Build history of the part. All positions in model axes, mm. A direction names the side the tool comes from. Give positions to 0.01 mm unless a question says otherwise; leave off trailing zeros. Loops run counter-clockwise (first coordinate to the right, second up) from the corner with the lowest first, then second, coordinate; pieces in that order, holes last. Notation, with made-up numbers: (-25.5, -30.5) -> (-9.5, -30.5) arc R13 ccw to (-9.5, -16.5) -> close; hole circle Ø6 at (13.5, -37). An arc over 180 degrees is marked (long way). Answer as a JSON object with one key per item and string values. Group by question number.
from build123d import *

# Parameters (mm, degrees)
SKETCH1_R                       = 4
BOSS_EXTRUDE1_DEPTH             = 45
SKETCH2_R                       = 1.625
BOSS_EXTRUDE2_DEPTH             = 2
FILLET1_R                       = 1
FILLET1_OF_MIRROR1_R            = 1
BOSS_EXTRUDE3_REACH             = 49.339
BOSS_EXTRUDE3_DIRECTION_2_REACH = 49.339
SKETCH5_W                       = 68.734952121
SKETCH5_H                       = 6.985
BOSS_EXTRUDE4_DEPTH             = 3.25
FILLET2_R                       = 3.175
FILLET3_R                       = 10
BOSS_EXTRUDE5_DEPTH             = 36.449
SKETCH7_W                       = 19.05
SKETCH7_H                       = 25.4
CUT_EXTRUDE1_DEPTH              = 33.782
FILLET4_R                       = 2
CUT_EXTRUDE2_DEPTH              = 134.693288074
CUT_EXTRUDE3_DEPTH              = 99.825981407
CUT_EXTRUDE3_DEPTH_BACK         = 99.825981407
SKETCH13_R                      = 1.625
SKETCH14_W                      = 22.869052137
SKETCH14_H                      = 20
CUT_EXTRUDE4_DEPTH              = 134.693288074
FILLET5_R                       = 1


with BuildPart() as part:
    # Sketch1 → Boss-Extrude1 (new, symmetric)
    with BuildSketch(Plane.XY):
        with Locations(Location((0, 0, 0), (0, 0, 180))):
            Circle(SKETCH1_R)
    extrude(amount=BOSS_EXTRUDE1_DEPTH, both=True)

    # Sketch2 → Boss-Extrude2 (add)
    with BuildSketch(Plane.XY.offset(45)):
        Circle(SKETCH2_R)
    boss_extrude2 = extrude(amount=BOSS_EXTRUDE2_DEPTH)

    # Fillet1
    fillet1_edges = [part.edges().sort_by_distance(p)[0] for p in [
        (-1.625, 0, 47),
    ]]
    fillet(fillet1_edges, radius=FILLET1_R)

    # Mirror1: Boss-Extrude2 across plane
    add(boss_extrude2.mirror(Plane.XY))

    # Fillet1 of Mirror1
    fillet1_of_mirror1_edges = [part.edges().sort_by_distance(p)[0] for p in [
        (-1.625, 0, -47),
    ]]
    fillet(fillet1_of_mirror1_edges, radius=FILLET1_OF_MIRROR1_R)

    # Boss-Extrude3: up to this face of the body (flat: up to its plane)
    boss_extrude3_end = Plane(part.part.faces().sort_by_distance((3.886862915, 0, 45))[0])
    # Sketch3 → Boss-Extrude3 (add, up to the picked face)
    with BuildSketch(Plane.XY, mode=Mode.PRIVATE) as boss_extrude3_sk1:
        Polygon((0, 0), (0, 1.625), (-74.93, 1.625), (-74.93, -1.625), (0, -1.625), align=None)
    boss_extrude3_tool1 = split(extrude(boss_extrude3_sk1.sketch, amount=BOSS_EXTRUDE3_REACH, mode=Mode.PRIVATE), bisect_by=boss_extrude3_end, keep=Keep.BOTH, mode=Mode.PRIVATE)
    add(boss_extrude3_tool1.solids().sort_by(Axis((-37.465, 0, 0), (0, 0, 1)))[0])

    # Boss-Extrude3 direction 2: up to this face of the body (flat: up to its plane)
    boss_extrude3_direction_2_end = Plane(part.part.faces().sort_by_distance((3.886862915, 0, -45))[0])
    # Sketch3 → Boss-Extrude3 direction 2 (add, up to the picked face)
    with BuildSketch(Plane.XY, mode=Mode.PRIVATE) as boss_extrude3_direction_2_sk1:
        Polygon((0, 0), (0, 1.625), (-74.93, 1.625), (-74.93, -1.625), (0, -1.625), align=None)
    boss_extrude3_direction_2_tool1 = split(extrude(boss_extrude3_direction_2_sk1.sketch, amount=-BOSS_EXTRUDE3_DIRECTION_2_REACH, mode=Mode.PRIVATE), bisect_by=boss_extrude3_direction_2_end, keep=Keep.BOTH, mode=Mode.PRIVATE)
    add(boss_extrude3_direction_2_tool1.solids().sort_by(Axis((-37.465, 0, 0), (0, 0, -1)))[0])

    # Sketch5 → Boss-Extrude4 (add)
    with BuildSketch(Plane(origin=(0, 1.625, 0), x_dir=(1, 0, 0), z_dir=(0, 1, 0))):
        with Locations((-40.56252394, 48.4925)):
            Rectangle(SKETCH5_W, SKETCH5_H)
    boss_extrude4 = extrude(amount=-BOSS_EXTRUDE4_DEPTH)

    # Mirror2: Boss-Extrude4 across plane
    add(boss_extrude4.mirror(Plane.XY))

    # Fillet2
    # the kernel refuses this fillet: 3.175 mm, written as the material it adds along each edge
    with BuildSketch(Plane(origin=(-6.195047879, 1.625, -45), x_dir=(1, 0, 0), z_dir=(0, -1, 0))) as fillet2_piece_1_section:
        with BuildLine():
            CenterArc((FILLET2_R, -FILLET2_R), FILLET2_R, 90, 90)
            Line((0, -FILLET2_R), (0, 0))
            Line((0, 0), (FILLET2_R, 0))
        make_face()
    fillet2_piece_1 = extrude(amount=3.25, mode=Mode.PRIVATE)
    fillet2_piece_1 = fillet2_piece_1 - Plane(origin=(0, 0, -45.745349648), x_dir=(-1, 0, 0), z_dir=(0, 0, 1)) * Cylinder(4, 20, mode=Mode.PRIVATE)
    add(fillet2_piece_1)
    with BuildSketch(Plane(origin=(-6.195047879, 9.5625, -45), x_dir=(1, 0, 0), z_dir=(0, -1, 0))) as fillet2_piece_2_section:
        with BuildLine():
            CenterArc((FILLET2_R, -FILLET2_R), FILLET2_R, 90, 90)
            Line((0, -FILLET2_R), (0, 0))
            Line((0, 0), (FILLET2_R, 0))
        make_face()
    fillet2_piece_2 = extrude(amount=11.1875, mode=Mode.PRIVATE)
    fillet2_piece_2 = split(fillet2_piece_2, bisect_by=Plane(origin=(-3.269448726, 1.625, -44.97522317), z_dir=(0, 1, 0)), keep=Keep.TOP, mode=Mode.PRIVATE)
    fillet2_piece_2 = fillet2_piece_2 & Plane(origin=(0, 0, -44.97522317), x_dir=(-1, 0, 0), z_dir=(0, 0, 1)) * Cylinder(4, 36, mode=Mode.PRIVATE)
    add(fillet2_piece_2)
    with BuildSketch(Plane(origin=(-6.195047879, 1.625, -45), x_dir=(1, 0, 0), z_dir=(0, -1, 0))) as fillet2_piece_3_section:
        with BuildLine():
            CenterArc((FILLET2_R, -FILLET2_R), FILLET2_R, 90, 90)
            Line((0, -FILLET2_R), (0, 0))
            Line((0, 0), (FILLET2_R, 0))
        make_face()
    fillet2_piece_3 = extrude(amount=3.25, mode=Mode.PRIVATE)
    fillet2_piece_3 = fillet2_piece_3 & Plane(origin=(0, 0, -44.99635319), x_dir=(-1, 0, 0), z_dir=(0, 0, 1)) * Cylinder(4, 20, mode=Mode.PRIVATE)
    add(fillet2_piece_3)
    with BuildSketch(Plane(origin=(-6.195047879, 1.625, -45), x_dir=(1, 0, 0), z_dir=(0, -1, 0))) as fillet2_piece_4_section:
        with BuildLine():
            CenterArc((FILLET2_R, -FILLET2_R), FILLET2_R, 90, 90)
            Line((0, -FILLET2_R), (0, 0))
            Line((0, 0), (FILLET2_R, 0))
        make_face()
    fillet2_piece_4 = extrude(amount=11.1875, mode=Mode.PRIVATE)
    fillet2_piece_4 = split(fillet2_piece_4, bisect_by=Plane(origin=(-3.269448726, -1.625, -44.97522317), z_dir=(0, -1, 0)), keep=Keep.TOP, mode=Mode.PRIVATE)
    fillet2_piece_4 = fillet2_piece_4 & Plane(origin=(0, 0, -44.97522317), x_dir=(-1, 0, 0), z_dir=(0, 0, 1)) * Cylinder(4, 36, mode=Mode.PRIVATE)
    add(fillet2_piece_4)
    with BuildSketch(Plane(origin=(-6.195047879, 1.625, 45), x_dir=(1, 0, 0), z_dir=(0, -1, 0))) as fillet2_piece_5_section:
        with BuildLine():
            CenterArc((FILLET2_R, FILLET2_R), FILLET2_R, 180, 90)
            Line((0, FILLET2_R), (0, 0))
            Line((0, 0), (FILLET2_R, 0))
        make_face()
    fillet2_piece_5 = extrude(amount=3.25, mode=Mode.PRIVATE)
    fillet2_piece_5 = fillet2_piece_5 - Plane(origin=(0, 0, 45.745349648), x_dir=(-1, 0, 0), z_dir=(0, 0, 1)) * Cylinder(4, 20, mode=Mode.PRIVATE)
    add(fillet2_piece_5)
    with BuildSketch(Plane(origin=(-6.195047879, 9.5625, 45), x_dir=(1, 0, 0), z_dir=(0, -1, 0))) as fillet2_piece_6_section:
        with BuildLine():
            CenterArc((FILLET2_R, FILLET2_R), FILLET2_R, 180, 90)
            Line((0, FILLET2_R), (0, 0))
            Line((0, 0), (FILLET2_R, 0))
        make_face()
    fillet2_piece_6 = extrude(amount=11.1875, mode=Mode.PRIVATE)
    fillet2_piece_6 = fillet2_piece_6 & Plane(origin=(0, 0, 44.97522317), x_dir=(-1, 0, 0), z_dir=(0, 0, 1)) * Cylinder(4, 36, mode=Mode.PRIVATE)
    fillet2_piece_6 = split(fillet2_piece_6, bisect_by=Plane(origin=(-3.269448726, 1.625, 44.97522317), z_dir=(0, 1, 0)), keep=Keep.TOP, mode=Mode.PRIVATE)
    add(fillet2_piece_6)
    with BuildSketch(Plane(origin=(-6.195047879, 1.625, 45), x_dir=(1, 0, 0), z_dir=(0, -1, 0))) as fillet2_piece_7_section:
        with BuildLine():
            CenterArc((FILLET2_R, FILLET2_R), FILLET2_R, 180, 90)
            Line((0, FILLET2_R), (0, 0))
            Line((0, 0), (FILLET2_R, 0))
        make_face()
    fillet2_piece_7 = extrude(amount=3.25, mode=Mode.PRIVATE)
    fillet2_piece_7 = fillet2_piece_7 & Plane(origin=(0, 0, 44.99635319), x_dir=(-1, 0, 0), z_dir=(0, 0, 1)) * Cylinder(4, 20, mode=Mode.PRIVATE)
    add(fillet2_piece_7)
    with BuildSketch(Plane(origin=(-6.195047879, 1.625, 45), x_dir=(1, 0, 0), z_dir=(0, -1, 0))) as fillet2_piece_8_section:
        with BuildLine():
            CenterArc((FILLET2_R, FILLET2_R), FILLET2_R, 180, 90)
            Line((0, FILLET2_R), (0, 0))
            Line((0, 0), (FILLET2_R, 0))
        make_face()
    fillet2_piece_8 = extrude(amount=11.1875, mode=Mode.PRIVATE)
    fillet2_piece_8 = fillet2_piece_8 & Plane(origin=(0, 0, 44.97522317), x_dir=(-1, 0, 0), z_dir=(0, 0, 1)) * Cylinder(4, 36, mode=Mode.PRIVATE)
    fillet2_piece_8 = split(fillet2_piece_8, bisect_by=Plane(origin=(-3.269448726, -1.625, 44.97522317), z_dir=(0, -1, 0)), keep=Keep.TOP, mode=Mode.PRIVATE)
    add(fillet2_piece_8)
    # the kernel refuses this fillet: 3.175 mm, written as the material it takes off along each edge
    with BuildSketch(Plane(origin=(-6.195047879, 9.5625, -51.985), x_dir=(0, 0, 1), z_dir=(0, -1, 0)), Plane(origin=(-6.195047879, 9.5625, 51.985), x_dir=(-1, 0, 0), z_dir=(0, -1, 0))) as fillet2_2_piece_1:
        with BuildLine():
            CenterArc((FILLET2_R, FILLET2_R), FILLET2_R, 180, 90)
            Line((0, FILLET2_R), (0, 0))
            Line((0, 0), (FILLET2_R, 0))
        make_face()
    extrude(amount=19.125, mode=Mode.SUBTRACT)

    # Fillet3
    fillet3_edges = [part.edges().sort_by_distance(p)[0] for p in [
        (-74.93, 0, -51.985),
        (-74.93, 0, 51.985),
    ]]
    fillet(fillet3_edges, radius=FILLET3_R)

    # Sketch6 → Boss-Extrude5 (add)
    with BuildSketch(Plane(origin=(0, 1.625, 0), x_dir=(1, 0, 0), z_dir=(0, 1, 0))):
        with BuildLine():
            Line((-9.370047879, 49.445), (-64.93, 49.445))
            ThreePointArc((-64.93, 49.445), (-70.205016588, 47.260016588), (-72.39, 41.985))
            Line((-72.39, 41.985), (-72.39, -41.985))
            ThreePointArc((-72.39, -41.985), (-70.205016588, -47.260016588), (-64.93, -49.445))
            Line((-64.93, -49.445), (-9.370047879, -49.445))
            Line((-9.370047879, -49.445), (-6.259195906, -49.445))
            ThreePointArc((-6.259195906, -49.445), (-7.362001565, -51.269344425), (-9.370047879, -51.985))
            Line((-9.370047879, -51.985), (-64.93, -51.985))
            ThreePointArc((-64.93, -51.985), (-72.001067812, -49.056067812), (-74.93, -41.985))
            Line((-74.93, -41.985), (-74.93, 41.985))
            ThreePointArc((-74.93, 41.985), (-72.001067812, 49.056067812), (-64.93, 51.985))
            Line((-64.93, 51.985), (-9.370047879, 51.985))
            ThreePointArc((-9.370047879, 51.985), (-7.362001565, 51.269344425), (-6.259195906, 49.445))
            Line((-6.259195906, 49.445), (-9.370047879, 49.445))
        make_face()
    extrude(amount=BOSS_EXTRUDE5_DEPTH)

    # Sketch7 → Cut-Extrude1 (cut)
    with BuildSketch(Plane.XZ.offset(1.625)):
        with Locations((-44.930047879, 28.085)):
            Rectangle(SKETCH7_W, SKETCH7_H)
    extrude(amount=-CUT_EXTRUDE1_DEPTH, mode=Mode.SUBTRACT)

    # Fillet4
    fillet4_edges = [part.edges().sort_by_distance(p)[0] for p in [
        (-35.405047879, 0, 40.785),
        (-35.405047879, 0, 15.385),
        (-54.455047879, 0, 15.385),
        (-54.455047879, 0, 40.785),
    ]]
    fillet(fillet4_edges, radius=FILLET4_R)

    # Sketch9 → Cut-Extrude2 (cut, through all)
    with BuildSketch(Plane(origin=(0, 0, -51.985), x_dir=(-1, 0, 0), z_dir=(0, 0, -1))):
        with BuildLine():
            Line((49.65002394, 8.074), (24.65002394, 8.074))
            ThreePointArc((24.65002394, 8.074), (14.65002394, 18.074), (24.65002394, 28.074))
            Line((24.65002394, 28.074), (49.65002394, 28.074))
            ThreePointArc((49.65002394, 28.074), (59.65002394, 18.074), (49.65002394, 8.074))
        make_face()
    extrude(amount=-CUT_EXTRUDE2_DEPTH, mode=Mode.SUBTRACT)

    # Sketch13 → Cut-Extrude3 (cut, two sides: drawn at the far end of the back side and taken through both)
    with BuildSketch(Plane.XY.offset(-CUT_EXTRUDE3_DEPTH_BACK)):
        Circle(SKETCH13_R)
    extrude(amount=CUT_EXTRUDE3_DEPTH + CUT_EXTRUDE3_DEPTH_BACK, mode=Mode.SUBTRACT)

    # Sketch14 → Cut-Extrude4 (cut, through all)
    with BuildSketch(Plane(origin=(0, 0, -51.985), x_dir=(-1, 0, 0), z_dir=(0, 0, -1))):
        with Locations((13.215497872, 18.074)):
            Rectangle(SKETCH14_W, SKETCH14_H)
    extrude(amount=-CUT_EXTRUDE4_DEPTH, mode=Mode.SUBTRACT)

    # Fillet5
    fillet5_edges = [part.edges().sort_by_distance(p)[0] for p in [
        (-53.869261442, 1.625, 40.199213562),
        (-44.930047879, 1.625, 40.785),
        (-35.990834317, 1.625, 40.199213562),
        (-35.405047879, 1.625, 28.085),
        (-35.990834317, 1.625, 15.970786438),
        (-44.930047879, 1.625, 15.385),
        (-53.869261442, 1.625, 15.970786438),
        (-53.869261442, -1.625, 40.199213562),
        (-44.930047879, -1.625, 40.785),
        (-35.990834317, -1.625, 40.199213562),
        (-35.405047879, -1.625, 28.085),
        (-35.990834317, -1.625, 15.970786438),
        (-44.930047879, -1.625, 15.385),
        (-53.869261442, -1.625, 15.970786438),
        (-37.15002394, 8.074, -49.445),
        (-59.65002394, 18.074, -49.445),
        (-37.15002394, 8.074, 49.445),
        (-59.65002394, 18.074, 49.445),
        (-59.65002394, 18.074, 51.985),
        (-37.15002394, 8.074, 51.985),
        (-54.455047879, 1.625, 28.085),
        (-54.455047879, -1.625, 28.085),
        (-37.15002394, 28.074, -49.445),
        (-37.15002394, 28.074, 49.445),
        (-37.15002394, 28.074, 51.985),
        (-7.362001565, 8.074, 51.269344425),
        (-7.362001565, 28.074, 51.269344425),
        (-6.259195906, 33.074, 49.445),
        (-6.259195906, 33.074, -49.445),
    ]]
    fillet(fillet5_edges, radius=FILLET5_R)


solid = part.part
(1) Probe line 1 along X through (y, z) = (0, 5) (3 decimals); line 2 along X through (y, z) = (0, 24.5) (3 decimals); line 3 along Y through (x, z) = (0, 18) (3 decimals). List the from-to ranges inside material, lowest first. Write a range as [from, to].
(2) Saw through at B-B on z = -12. List the corners of the cut face in (x, y) (3 decimals).
(3) Saw through at A-A on x = 0. List the corners of the cut face in (y, z) (3 decimals).
(4) Pull direction Z, two halves, no side cores. Call faces 5 (the cylindrical face through (-70.263, 19.594, 47.202)), 6 (the flat face through (1, 2, -45)), 7 (the flat face through (-74.93, 18, 1)): pulls with the +Z half, pulls with the -Z half, needs draft (parallel to the pull), parting line crosses it, or undercut.
(5) Saw through at C-C on x = -40. Give the number of separate pieces and of enclosed holes in the cut face, plus the area to 3 significant figures.
(6) Pin check, flat tips, straight feed: pin 1 (12 mm diameter, centred on x = -45, z = 39, fed in from -Y) (3 decimals); pin 2 (4 mm diameter, centred on x = -20, z = 41, fed in from +Y) (3 decimals); pin 3 (18 mm diameter, centred on x = -41.5, y = 24, fed in from +Z) (3 decimals); pin 4 (3.5 mm diameter, centred on x = -0.5, y = -1.5, fed in from -Z). Stop position of each tip, or through.
(7) Saw through at D-D on y = 33. List the corners of the cut face in (x, z) (3 decimals), plus the area to 3 significant figures.
(8) 3-axis set-ups, long thin cutter, end or side, ignore diameter. For faces 1 (the flat face through (-39, -1.625, 1)), 2 (the flat face through (-38, 1.625, 1)), 3 (the flat face through (-43, 32, 49.445)), 4 (the flat face through (1, 2, 45)): which of +Z, -Z, +X, -X, +Y, -Y reach the whole face in a straight line?
Calculated:
{
 "1": {"line 1": "x = [-74.93, -1.625], [1.625, 4]", "line 2": "x = [-74.93, -54.455], [-35.405, -1.625], [1.625, 4]", "line 3": "y = [-4, -1.625], [1.625, 4]"},
 "2": {"outline": "(-74.93, -1.625) -> (-3.655, -1.625) arc R4 ccw (long way) to (-3.655, 1.625) -> (-72.39, 1.625) -> (-72.39, 38.074) -> (-74.93, 38.074) -> close; hole circle Ø3.25 at (0, 0)"},
 "3": {"outline": "(-4, -45) -> (-1.625, -45) -> (-1.625, 45) -> (-4, 45) -> close; (1.625, -45) -> (4, -45) -> (4, 45) -> (1.625, 45) -> close"},
 "4": {"face 5": "undercut", "face 6": "pulls with the -Z half", "face 7": "needs draft"},
 "5": {"separate pieces": "4", "enclosed holes": "0", "area": "337 mm^2"},
 "6": {"pin 1": "stops at y = -1.625", "pin 2": "stops at y = 1.625", "pin 3": "stops at z = 51.985", "pin 4": "stops at z = -45"},
 "7": {"outline": "(-74.93, -41.985) arc R10 ccw to (-64.93, -51.985) -> (-9.37, -51.985) arc R3.175 ccw to (-7.276, -51.197) arc R1 ccw to (-7.936, -49.445) -> (-64.93, -49.445) arc R7.46 cw to (-72.39, -41.985) -> (-72.39, 41.985) arc R7.46 cw to (-64.93, 49.445) -> (-7.936, 49.445) arc R1 ccw to (-7.276, 51.197) arc R3.175 ccw to (-9.37, 51.985) -> (-64.93, 51.985) arc R10 ccw to (-74.93, 41.985) -> close", "area": "575 mm^2"},
 "8": {"face 1": "+Z, -Z, -X, -Y", "face 2": "+Y", "face 3": "+X, +Y", "face 4": "+Z, +X, +Y, -Y"}
}
